Verification items for this drawing (mm, ordinates from the low corner). A direction names the side the tool comes from. Round coordinates to 2 decimals unless told otherwise and drop trailing zeros. Order: outer loops, then holes, each group sorted by start corner. A loop starts at its lowest first (then second) coordinate and runs counter-clockwise, first axis right, second up. Notation, with made-up numbers: (-32.75, -17) -> (14.25, -17) arc R9 ccw to (14.25, -6) -> close; hole circle Ø1 at (51, 70.5). An arc over 180 degrees is marked (long way). Put each result on its own line as item: value.
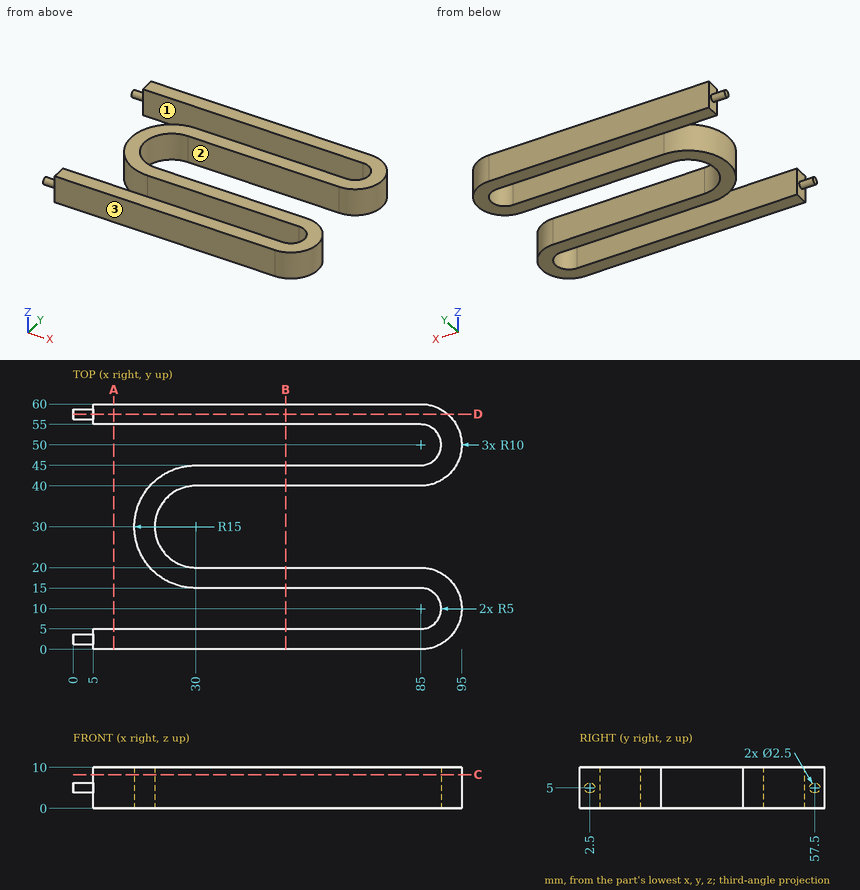
Item 1: Gauge pin test, flat ends, axial feed: pin 1 Ø2 at (y, z) = (34.5, 4) entering from -X; pin 2 Ø1 at (y, z) = (51.5, 8.5) entering from +X. Record the tip position at first contact, or that the pin passes through.
Check sheet entries:
pin 1: stops at x = 15.41
pin 2: stops at x = 94.95
Item 2: Material ranges on L1, parallel to Y at x = 36, z = 8; L2, parallel to Y at x = 27, z = 7.25; L3, parallel to Y at x = 14.5, z = 1, recorded low to high. Write a range as [from, to].
Check sheet entries:
L1: y = [0, 5], [15, 20], [40, 45], [55, 60]
L2: y = [0, 5], [15.3, 20.46], [39.54, 44.7], [55, 60]
L3: y = [0, 5], [55, 60]
Item 3: Section check A-A on x = 10. Record the boundary of the cut face in (y, z).
Check sheet entries:
outline: (0, 0) -> (5, 0) -> (5, 10) -> (0, 10) -> close; (55, 0) -> (60, 0) -> (60, 10) -> (55, 10) -> close
Item 4: Tool access check on the marked faces 1, 2 and 3. Record the directions out of +Z, -Z, +X, -X, +Y, -Y that give a thin tool (end or side, any length) a straight path to the whole face; none if there is none.
Check sheet entries:
face 1: +Z, -Z, -X
face 2: +Z, -Z, +X
face 3: +Z, -Z, +X, -X, -Y
Item 5: Section check D-D on y = 57.5. Record the boundary of the cut face in (x, z), then the cut area to 3 significant figures.
Check sheet entries:
outline: (0, 3.75) -> (5, 3.75) -> (5, 0) -> (91.61, 0) -> (91.61, 10) -> (5, 10) -> (5, 6.25) -> (0, 6.25) -> close
area: 879 mm^2
Item 6: Section check B-B on x = 52. Record the boundary of the cut face in (y, z), then the cut area to 3 significant figures.
Check sheet entries:
outline: (0, 0) -> (5, 0) -> (5, 10) -> (0, 10) -> close; (15, 0) -> (20, 0) -> (20, 10) -> (15, 10) -> close; (40, 0) -> (45, 0) -> (45, 10) -> (40, 10) -> close; (55, 0) -> (60, 0) -> (60, 10) -> (55, 10) -> close
area: 200 mm^2
Item 7: Section check C-C on z = 8.25. Record the boundary of the cut face in (x, y).
Check sheet entries:
outline: (5, 0) -> (85, 0) arc R10 ccw to (85, 20) -> (30, 20) arc R10 cw to (30, 40) -> (85, 40) arc R10 ccw to (85, 60) -> (5, 60) -> (5, 55) -> (85, 55) arc R5 cw to (85, 45) -> (30, 45) arc R15 ccw to (30, 15) -> (85, 15) arc R5 cw to (85, 5) -> (5, 5) -> close
